Verification items for this drawing (mm, ordinates from the low corner). Round coordinates to 2 decimals unless told otherwise and drop trailing zeros. Loops run counter-clockwise (first coordinate to the right, second up) from the corner with the lowest first, then second, coordinate; pieces in that order, holes last. Notation, with made-up numbers: M 3.25,-34.75 L 38.25,-34.75 A14 cw 38.25,-14.75 Z; hole C -17.75,-34.75 d1. An arc over 180 degrees is marked long. Write item = value, one per line. Start each with the question number.
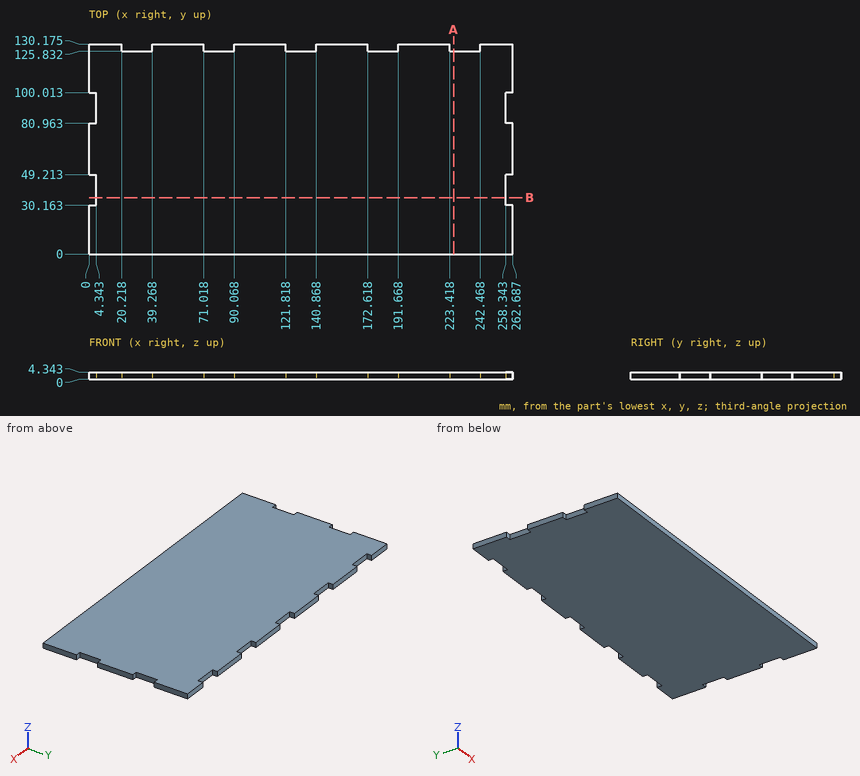
1. Thickness scan on line 1 (Y direction, x = 178, z = 1.3); line 2 (X direction, y = 86, z = 3.05). Record the ranges inside material, lowest first.
2. Gauge pin test, flat end, axial feed: P1, Ø1.3, axis at y = 94, z = 2, coming from the -X side. Record the tip position at first contact, or that the pin passes through.
3. Section check B-B, the plane y = 35. Enter the section's corners in (x, z).
4. Section check A-A, the plane x = 226. Enter the section's corners in (y, z).
Computed values:
q1.line_1 = 0 to 125.83
q1.line_2 = 4.34 to 258.34
q2.P1 = 4.34
q3.outline = M 4.34,0 L 258.34,0 L 258.34,4.34 L 4.34,4.34 Z
q4.outline = M 0,0 L 125.83,0 L 125.83,4.34 L 0,4.34 Z
